The model under review builds one solid part; all positions refer to its coordinate system, in mm. Round coordinates to 2 decimals unless told otherwise and drop trailing zeros. Write each loop counter-clockwise with the first axis right and the second up, starting at its lowest first coordinate (ties: lowest second). Pieces come first, ordered by that corner, then holes. Notation, with made-up numbers: (81, 14.25) - (85, 14.25) arc R24 ccw to (85, 28.25) - close; hole circle Ø5 at (-16.75, 75.25). An arc over 180 degrees is marked (long way). Use one line per item in the form item = value.
from build123d import *

# Parameters (mm, degrees)
SKETCH2_R           = 1.499999048
SKETCH2_R_2         = 8.476232568
BOSS_EXTRUDE1_DEPTH = 2
SKETCH3_R           = 2.000000571
BOSS_EXTRUDE4_DEPTH = 20
SKETCH5_R           = 1.499999048
SKETCH5_R_2         = 8.476232568
BOSS_EXTRUDE5_DEPTH = 2
SKETCH6_R           = 10.130319586
SKETCH6_R_2         = 8.476232568
BOSS_EXTRUDE6_DEPTH = 20


with BuildPart() as part:
    # Sketch2 → Boss-Extrude1 (new body)
    with BuildSketch(Plane.XY):
        Polygon((-1.529977411, 48.635467476), (1.529978834, 48.635467476), (42.884606582, -22.992698001), (41.354559362, -25.642734021), (-41.354559362, -25.642734021), (-42.884539813, -22.992735729), align=None)
        with Locations((-39.824585131, -22.992733702)):
            Circle(SKETCH2_R, mode=Mode.SUBTRACT)
        Circle(SKETCH2_R_2, mode=Mode.SUBTRACT)
        with Locations((1.077e-06, 45.98546927)):
            Circle(SKETCH2_R, mode=Mode.SUBTRACT)
        with Locations((39.824584054, -22.992735568)):
            Circle(SKETCH2_R, mode=Mode.SUBTRACT)
        with BuildLine():
            Line((8.625743911, -8.444177918), (6.753395324, -7.344905536))
            ThreePointArc((6.753395324, -7.344905536), (-0.619839897, -9.958503112), (-7.612069336, -6.450766323))
            Line((-7.612069336, -6.450766323), (-17.483000044, -7.749839951))
            ThreePointArc((-17.483000044, -7.749839951), (-18.685453818, -7.204965543), (-18.728632678, -5.885526729))
            Line((-18.728632678, -5.885526729), (-2.199572243, 22.743645745))
            ThreePointArc((-2.199572243, 22.743645745), (-2.657104073, 24.45117778), (-4.364636107, 23.99364595))
            Line((-4.364636107, 23.99364595), (-28.480761019, -17.776707679))
            ThreePointArc((-28.480761019, -17.776707679), (-28.480761019, -19.776707679), (-26.748710212, -20.776707679))
            Line((-26.748710212, -20.776707679), (29.264627025, -20.776707679))
            ThreePointArc((29.264627025, -20.776707679), (30.514626764, -19.52670794), (29.264627025, -18.276708201))
            Line((29.264627025, -18.276708201), (-22.096788511, -18.276708201))
            ThreePointArc((-22.096788511, -18.276708201), (-22.980671746, -17.910592355), (-23.34678825, -17.026709393))
            Line((-23.34678825, -17.026709393), (-23.34678825, -12.026708573))
            ThreePointArc((-23.34678825, -12.026708573), (-22.980671803, -11.142825281), (-22.096788511, -10.776708834))
            Line((-22.096788511, -10.776708834), (8.000743575, -10.776708834))
            ThreePointArc((8.000743575, -10.776708834), (9.201417559, -9.848429046), (8.625743911, -8.444177918))
        make_face(mode=Mode.SUBTRACT)
        with BuildLine():
            Line((-18.596788868, -15.776708722), (29.635460955, -15.776708722))
            ThreePointArc((29.635460955, -15.776708722), (31.367511763, -14.776708722), (31.367511763, -12.776708722))
            Line((31.367511763, -12.776708722), (3.360843145, 35.732264275))
            ThreePointArc((3.360843145, 35.732264275), (1.653311746, 36.189795934), (1.195780087, 34.482264536))
            Line((1.195780087, 34.482264536), (26.876487855, -9.998026092))
            ThreePointArc((26.876487855, -9.998026092), (27.00136385, -10.946549351), (26.418957002, -11.705557025))
            Line((26.418957002, -11.705557025), (22.088829273, -14.205557435))
            ThreePointArc((22.088829273, -14.205557435), (21.140305665, -14.330432937), (20.381297875, -13.748025775))
            Line((20.381297875, -13.748025775), (5.332531832, 12.317201602))
            ThreePointArc((5.332531832, 12.317201602), (3.928280962, 12.89287588), (3.000000636, 11.692202312))
            Line((3.000000636, 11.692202312), (2.984177121, 9.52106468))
            ThreePointArc((2.984177121, 9.52106468), (8.934236627, 4.442454459), (9.392562178, -3.366862259))
            Line((9.392562178, -3.366862259), (15.453058295, -11.265802197))
            ThreePointArc((15.453058295, -11.265802197), (15.582410103, -12.579594916), (14.461332001, -13.276708312))
            Line((14.461332001, -13.276708312), (-18.596788868, -13.276708312))
            ThreePointArc((-18.596788868, -13.276708312), (-19.846789073, -14.526708517), (-18.596788868, -15.776708722))
        make_face(mode=Mode.SUBTRACT)
        with BuildLine():
            Line((-32.625470169, -14.955556596), (-4.618801551, 33.553416401))
            ThreePointArc((-4.618801551, 33.553416401), (-2.886750744, 34.553416401), (-1.154699936, 33.553416401))
            Line((-1.154699936, 33.553416401), (22.961424976, -8.216937228))
            ThreePointArc((22.961424976, -8.216937228), (22.503893146, -9.924469262), (20.796361111, -9.466937433))
            Line((20.796361111, -9.466937433), (4.267300677, 19.162235041))
            ThreePointArc((4.267300677, 19.162235041), (3.103043715, 19.78456046), (2.029941749, 19.015642148))
            Line((2.029941749, 19.015642148), (-1.780492842, 9.817628582))
            ThreePointArc((-1.780492842, 9.817628582), (-8.31439673, 5.516048653), (-9.737572444, -2.176159144))
            Line((-9.737572444, -2.176159144), (-11.625744547, -3.248024394))
            ThreePointArc((-11.625744547, -3.248024394), (-13.12969852, -3.044446834), (-13.333275407, -1.540492769))
            Line((-13.333275407, -1.540492769), (1.715490636, 24.524734609))
            ThreePointArc((1.715490636, 24.524734609), (1.840366138, 25.473258218), (1.257958977, 26.232266008))
            Line((1.257958977, 26.232266008), (-3.072168752, 28.732266418))
            ThreePointArc((-3.072168752, 28.732266418), (-4.020692104, 28.857141706), (-4.779699344, 28.274734293))
            Line((-4.779699344, 28.274734293), (-30.460407112, -16.205556335))
            ThreePointArc((-30.460407112, -16.205556335), (-32.16793851, -16.663087995), (-32.625470169, -14.955556596))
        make_face(mode=Mode.SUBTRACT)
    extrude(amount=BOSS_EXTRUDE1_DEPTH)

    # Sketch3 → Boss-Extrude4 (add)
    with BuildSketch(Plane.XY.offset(2)):
        with Locations((-35.383429378, -20.428633317)):
            Circle(SKETCH3_R)
        with Locations((35.383430107, -20.428632056)):
            Circle(SKETCH3_R)
        with Locations((-7.28e-07, 40.857265373)):
            Circle(SKETCH3_R)
    extrude(amount=BOSS_EXTRUDE4_DEPTH)

    # Sketch5 → Boss-Extrude5 (add)
    with BuildSketch(Plane.XY.offset(22)):
        Polygon((-1.529977411, 48.635467476), (1.529978834, 48.635467476), (42.884606582, -22.992698001), (41.354559362, -25.642734021), (-41.354559362, -25.642734021), (-42.884539813, -22.992735729), align=None)
        with Locations(Location((-39.824585103, -22.992733751, 0), (0, 0, 1.842e-06))):
            Circle(SKETCH5_R, mode=Mode.SUBTRACT)
        Circle(SKETCH5_R_2, mode=Mode.SUBTRACT)
        with Locations((1.021e-06, 45.98546927)):
            Circle(SKETCH5_R, mode=Mode.SUBTRACT)
        with Locations(Location((39.824584082, -22.992735519, 0), (0, 0, 359.999998157))):
            Circle(SKETCH5_R, mode=Mode.SUBTRACT)
        with BuildLine():
            Line((8.625743911, -8.444177918), (6.753395324, -7.344905536))
            ThreePointArc((6.753395324, -7.344905536), (-0.619839897, -9.958503112), (-7.612069336, -6.450766323))
            Line((-7.612069336, -6.450766323), (-17.483000044, -7.749839951))
            ThreePointArc((-17.483000044, -7.749839951), (-18.685453818, -7.204965543), (-18.728632678, -5.885526729))
            Line((-18.728632678, -5.885526729), (-2.199572243, 22.743645745))
            ThreePointArc((-2.199572243, 22.743645745), (-2.657104073, 24.45117778), (-4.364636107, 23.99364595))
            Line((-4.364636107, 23.99364595), (-28.480761019, -17.776707679))
            ThreePointArc((-28.480761019, -17.776707679), (-28.480761019, -19.776707679), (-26.748710212, -20.776707679))
            Line((-26.748710212, -20.776707679), (29.264627025, -20.776707679))
            ThreePointArc((29.264627025, -20.776707679), (30.514626764, -19.52670794), (29.264627025, -18.276708201))
            Line((29.264627025, -18.276708201), (-22.096790373, -18.276708201))
            ThreePointArc((-22.096790373, -18.276708201), (-22.980673007, -17.910592026), (-23.346789181, -17.026709393))
            Line((-23.346789181, -17.026709393), (-23.346789181, -12.026708573))
            ThreePointArc((-23.346789181, -12.026708573), (-22.980672734, -11.142825281), (-22.096789442, -10.776708834))
            Line((-22.096789442, -10.776708834), (8.000743575, -10.776708834))
            ThreePointArc((8.000743575, -10.776708834), (9.201417559, -9.848429046), (8.625743911, -8.444177918))
        make_face(mode=Mode.SUBTRACT)
        with BuildLine():
            Line((-18.596788868, -15.776708722), (29.635460955, -15.776708722))
            ThreePointArc((29.635460955, -15.776708722), (31.367511763, -14.776708722), (31.367511763, -12.776708722))
            Line((31.367511763, -12.776708722), (3.360843145, 35.732264275))
            ThreePointArc((3.360843145, 35.732264275), (1.653311746, 36.189795934), (1.195780087, 34.482264536))
            Line((1.195780087, 34.482264536), (26.876488786, -9.998027705))
            ThreePointArc((26.876488786, -9.998027705), (27.001364195, -10.946550607), (26.418957468, -11.705557831))
            Line((26.418957468, -11.705557831), (22.088829739, -14.205558241))
            ThreePointArc((22.088829739, -14.205558241), (21.14030613, -14.330433743), (20.38129834, -13.748026582))
            Line((20.38129834, -13.748026582), (5.332531832, 12.317201602))
            ThreePointArc((5.332531832, 12.317201602), (3.928280962, 12.89287588), (3.000000636, 11.692202312))
            Line((3.000000636, 11.692202312), (2.984177121, 9.52106468))
            ThreePointArc((2.984177121, 9.52106468), (8.934236627, 4.442454459), (9.392562178, -3.366862259))
            Line((9.392562178, -3.366862259), (15.453058295, -11.265802197))
            ThreePointArc((15.453058295, -11.265802197), (15.582410103, -12.579594916), (14.461332001, -13.276708312))
            Line((14.461332001, -13.276708312), (-18.596788868, -13.276708312))
            ThreePointArc((-18.596788868, -13.276708312), (-19.846789073, -14.526708517), (-18.596788868, -15.776708722))
        make_face(mode=Mode.SUBTRACT)
        with BuildLine():
            Line((-32.625470169, -14.955556596), (-4.618801551, 33.553416401))
            ThreePointArc((-4.618801551, 33.553416401), (-2.886750744, 34.553416401), (-1.154699936, 33.553416401))
            Line((-1.154699936, 33.553416401), (22.961424976, -8.216937228))
            ThreePointArc((22.961424976, -8.216937228), (22.503893146, -9.924469262), (20.796361111, -9.466937433))
            Line((20.796361111, -9.466937433), (4.267300677, 19.162235041))
            ThreePointArc((4.267300677, 19.162235041), (3.103043715, 19.78456046), (2.029941749, 19.015642148))
            Line((2.029941749, 19.015642148), (-1.780492842, 9.817628582))
            ThreePointArc((-1.780492842, 9.817628582), (-8.31439673, 5.516048653), (-9.737572444, -2.176159144))
            Line((-9.737572444, -2.176159144), (-11.625744547, -3.248024394))
            ThreePointArc((-11.625744547, -3.248024394), (-13.12969852, -3.044446834), (-13.333275407, -1.540492769))
            Line((-13.333275407, -1.540492769), (1.715491102, 24.524735416))
            ThreePointArc((1.715491102, 24.524735416), (1.840366604, 25.473259024), (1.257959442, 26.232266814))
            Line((1.257959442, 26.232266814), (-3.072168286, 28.732267224))
            ThreePointArc((-3.072168286, 28.732267224), (-4.020691188, 28.857142633), (-4.779698413, 28.274735906))
            Line((-4.779698413, 28.274735906), (-30.460407112, -16.205556335))
            ThreePointArc((-30.460407112, -16.205556335), (-32.16793851, -16.663087995), (-32.625470169, -14.955556596))
        make_face(mode=Mode.SUBTRACT)
    extrude(amount=BOSS_EXTRUDE5_DEPTH)

    # Sketch6 → Boss-Extrude6 (add)
    with BuildSketch(Plane.XY.offset(24)):
        with Locations(Location((0, 0, 0), (0, 0, 192.86084428))):
            Circle(SKETCH6_R)
        Circle(SKETCH6_R_2, mode=Mode.SUBTRACT)
    extrude(amount=BOSS_EXTRUDE6_DEPTH)


solid = part.part
(1) Insertion check: P1, Ø13.5, axis at x = 0, y = 0, coming from the -Z side (1 decimal); P2, Ø1, axis at x = -8, z = 23.5, coming from the +Y side; P3, Ø4, axis at x = -39.82, y = -22.99, coming from the +Z side; P4, Ø1.6, axis at x = 4.5, z = 1, coming from the +Y side. Each pin has a flat end and moves straight along its axis. Give the tip position at first contact, or say it passes through.
Geometry results:
P1 = through
P2 = 38.3
P3 = 24
P4 = 44.88
(2) The part is to be moulded in two halves that separate along Y. For faces 1 (the cylindrical face through (3.95, 12.9, 0.99)), 2 (the flat face through (-22.497, 12.32, 0.986)), say which applies: +Y half, -Y half, draft (parallel to the pull), parting line (faces both ways), or undercut.
Geometry results:
face_1 = undercut
face_2 = +Y half
(3) Add section A-A on x = 24.5. Count the separate pieces of the cut face and the enclosed holes in it, then the cut area to 3 significant figures.
Geometry results:
separate_pieces = 8
enclosed_holes = 0
area = 96.1 mm2
(4) To check wall thickness, follow L1, parallel to Z at x = -4, y = 35; L2, parallel to Y at x = 0, z = 26.5; L3, parallel to Z at x = 3.5, y = 9. State the ranges of each line that lie inside material, in increasing order.
Geometry results:
L1 = 0 to 2, 22 to 24
L2 = -10.13 to -8.48, 8.48 to 10.13
L3 = 0 to 2, 22 to 44
(5) Add section C-C on z = 14.5. Write out the cut boundary in (x, y).
Geometry results:
outline = circle Ø4 at (-35.38, -20.43); circle Ø4 at (0, 40.86); circle Ø4 at (35.38, -20.43)
